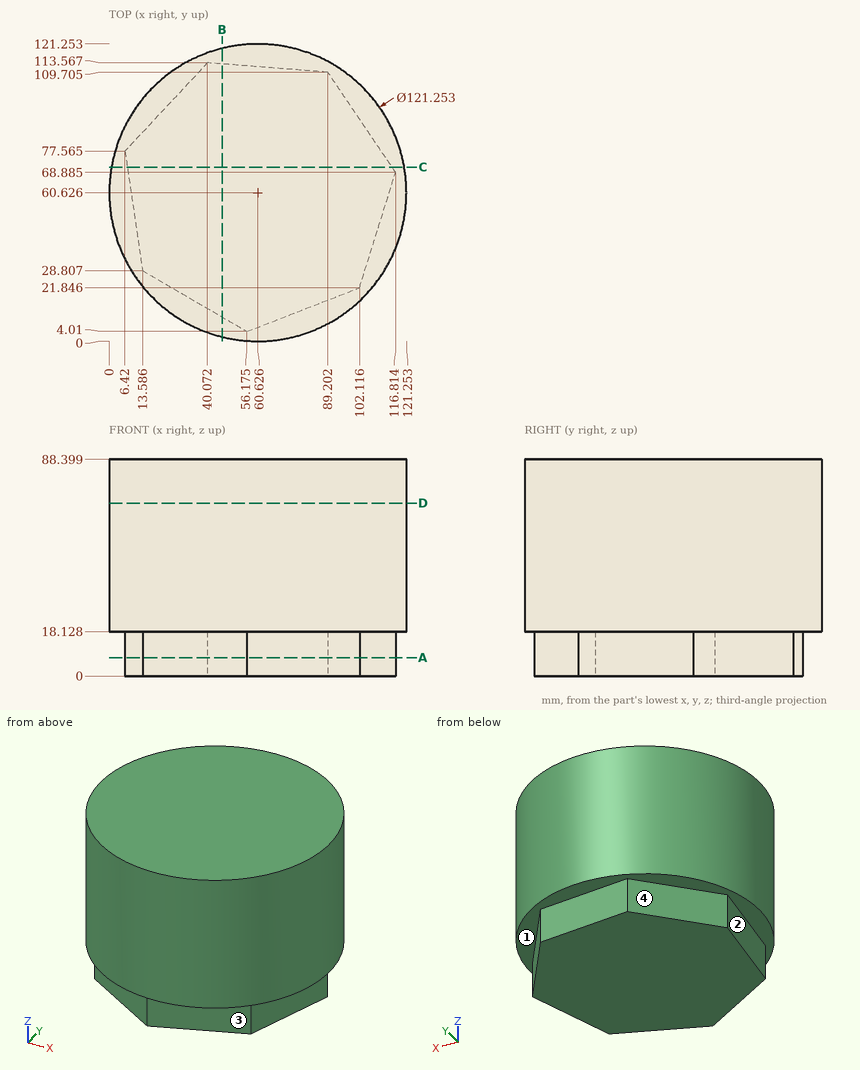
Answer from the drawing. Dimensions are ordinates in mm from the lowest x, y and z of the part. A direction names the side the tool comes from. Give positions to 0.01 mm unless a question says otherwise; leave off trailing zeros. Order: outer loops, then holes, each group sorted by start corner. A loop starts at its lowest first (then second) coordinate and runs counter-clockwise, first axis right, second up. Notation, with made-up numbers: (-10.5, 28) -> (43.5, 28) arc R28 cw to (43.5, 58) -> close; hole circle Ø3 at (64.5, 37.5). An arc over 180 degrees is marked (long way). One line per item, written item: value.
Item 1: Find section A-A, the plane z = 7.5. Give the vertices of the cut face in (x, y) (1 decimal).
Answer sheet:
outline: (6.4, 77.6) -> (13.6, 28.8) -> (56.2, 4) -> (102.1, 21.8) -> (116.8, 68.9) -> (89.2, 109.7) -> (40.1, 113.6) -> close
Item 2: Flat-ended cylindrical pins translate along their axes: P1, Ø2, axis at x = 23, z = 70, coming from the +Y side; P2, Ø10, axis at y = 95.5, z = 37.5, coming from the -X side; P3, Ø3, axis at x = 43, z = 28.5, coming from the -Y side (1 decimal). Find the tip coordinate at first contact, or state that the pin passes through.
Answer sheet:
P1: y = 108.94
P2: x = 7.87
P3: y = 2.2
Item 3: Find section C-C, the plane y = 71. Give the vertices of the cut face in (x, z) (1 decimal), plus the area to 3 significant figures.
Answer sheet:
outline: (0.9, 18.1) -> (7.4, 18.1) -> (7.4, 0) -> (115.4, 0) -> (115.4, 18.1) -> (120.4, 18.1) -> (120.4, 88.4) -> (0.9, 88.4) -> close
area: 10,400 mm²
Item 4: A tool of negligible diameter and unlimited length cuts with its end or side. For the marked faces 1, 2, 3 and 4, from which of +Z, -Z, +X, -X, +Y, -Y can it reach the whole face along a straight path? Write none if from no direction.
Answer sheet:
face 1: -Z
face 2: -Z, -X, -Y
face 3: -Z, +X, -Y
face 4: -Z, -X, +Y
Item 5: Find section D-D, the plane z = 70.5. Give the vertices of the cut face in (x, y), plus the area to 3 significant figures.
Answer sheet:
outline: circle Ø121.25 at (60.63, 60.63)
area: 11,500 mm²
Item 6: Straight lines are drawn through the part: probe 1 along X at (y, z) = (62.5, 33.5); probe 2 along X at (y, z) = (39, 25.5) (1 decimal); probe 3 along Z at (x, y) = (31, 8.5). For each, find the intervals that lie inside material, in ascending order.
Answer sheet:
probe 1: 0.03 to 121.22
probe 2: 4 to 117.3
probe 3: 18.13 to 88.4
Item 7: Find section B-B, the plane x = 46. Give the vertices of the cut face in (y, z) (1 decimal), plus the area to 3 significant figures.
Answer sheet:
outline: (1.8, 18.1) -> (9.9, 18.1) -> (9.9, 0) -> (113.1, 0) -> (113.1, 18.1) -> (119.5, 18.1) -> (119.5, 88.4) -> (1.8, 88.4) -> close
area: 10,100 mm²
